Check sheet for the drawn part. Datum: minimum x, y, z corner. Units: mm. A direction names the side the tool comes from. Give positions to 0.01 mm unless a question says otherwise; leave off trailing zeros. Loops run counter-clockwise (first coordinate to the right, second up) from the corner with the lowest first, then second, coordinate; pieces in that order, holes last.
1. Cross-section at B-B, the plane z = 4.25. Record the cut outline in (x, y).
2. Tool access check on the marked faces 1 and 2. Record the directions out of +Z, -Z, +X, -X, +Y, -Y that give a thin tool (end or side, any length) a straight path to the whole face; none if there is none.
3. Material ranges on L1, parallel to Z at x = 0.75, y = 3.25 (1 decimal); L2, parallel to Y at x = 6.5, z = 8; L3, parallel to X at y = 6, z = 17, recorded low to high.
4. Go/stop test with flat-tipped pins: pin 1 Ø2 at (x, z) = (5, 2.5) entering from +Y; pin 2 Ø1.5 at (x, y) = (7.5, 8.5) entering from -Z; pin 3 Ø1.5 at (y, z) = (3.5, 15) entering from -X. Record where each tip stops, or that it passes through.
5. Cross-section at A-A, the plane y = 4.75. Record the cut outline in (x, z).
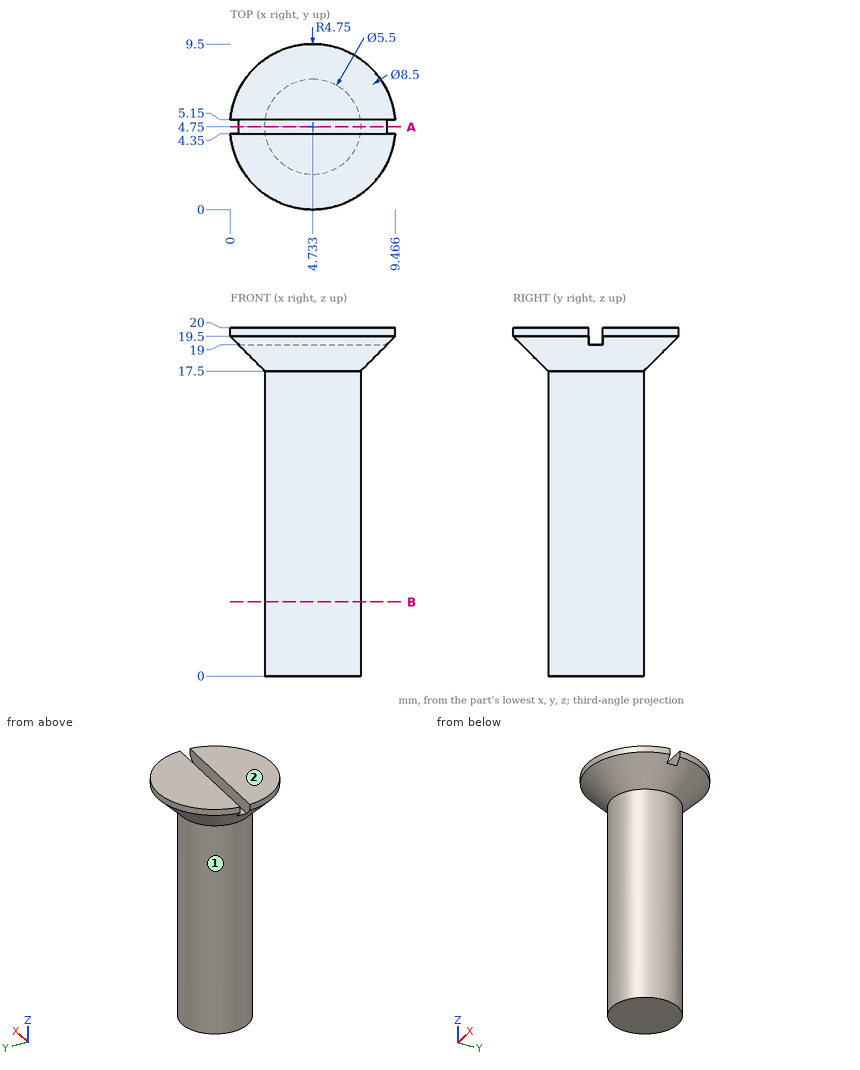
Result:
1. outline: circle Ø5.5 at (4.73, 4.75)
2. face 1: -Z
2. face 2: +Z, +X, -X, +Y, -Y
3. L1: z = 19 to 20
3. L2: y = 2.64 to 6.86
3. L3: x = 2.28 to 7.18
4. pin 1: stops at y = 7.5
4. pin 2: stops at z = 18.66
4. pin 3: stops at x = 2.03
5. outline: (0.48, 19) - (1.98, 17.5) - (1.98, 0) - (7.48, 0) - (7.48, 17.5) - (8.98, 19) - close
